The model under review builds one solid part; all positions refer to its coordinate system, in mm. Face numbers are marked on the shaded views. A direction names the side the tool comes from. Round coordinates to 2 decimals unless told otherwise and drop trailing zeros. Write each loop counter-clockwise with the first axis right and the second up, starting at its lowest first coordinate (ties: lowest second). Pieces come first, ordered by that corner, then holes. Notation, with made-up numbers: M 49.5,20.5 L 91.5,20.5 A31 cw 91.5,56.5 Z; hole C 45.25,-15.75 d9. An arc over 180 degrees is marked long. One line per item, written item: value. Start each with the question number.
1) Take a section at A-A, the plane x = 30. Write out the cut boundary in (y, z).
2) Wall thickness on probe 1 along Y at (x, z) = (0, 1.5); probe 2 along X at (y, z) = (-17.5, 0.5); probe 3 along X at (y, z) = (41.5, 0.75): over which ranges is each line inside the solid? List them lowest first.
3) Tool access review of the marked faces 4 and 5: name each direction out of +Z, -Z, +X, -X, +Y, -Y from which nothing blocks a thin tool from reaching the whole face with its end or side.
4) Take a section at B-B, the plane y = 20. Write out the cut boundary in (x, z), and give its area (3 significant figures).
5) Mouldability with a two-part tool opening along Y and no side actions: class the marked faces 1, 2 and 3 as +Y half, -Y half, draft (parallel to the pull), parting line (faces both ways), or undercut.
6) For P1, Ø2.5, axis at x = -66.82, y = 3.94, coming from the +Z side; P2, Ø4, axis at y = 53.5, z = 6.5, coming from the +X side; P3, Ø1.5, axis at x = 48.5, y = -28.5, coming from the +Z side; P4, Ø4, axis at x = 45, z = 4.5, coming from the -Y side, all flat-tipped, find the tip position at first contact; note any pin that passes through.
from build123d import *

# Parameters (mm, degrees)
BOSS_EXTRUDE1_DEPTH = 8
SKETCH2_R           = 2.25
CUT_EXTRUDE1_DEPTH  = 28
FILLET1_R           = 10
SKETCH5_R           = 1.65
CUT_EXTRUDE3_DEPTH  = 45
SKETCH10_R          = 4
CUT_EXTRUDE4_DEPTH  = 5
CUT_EXTRUDE5_DEPTH  = 10
CHAMFER1_SIZE       = 8.908764189
CHAMFER1_SIZE_2     = 10
CHAMFER1_SIZE_3     = 8.898783464
SKETCH12_R          = 10
CUT_EXTRUDE6_DEPTH  = 25.5
SKETCH13_R          = 1.65
CUT_EXTRUDE7_DEPTH  = 10
SKETCH14_R          = 2.55
CUT_EXTRUDE8_DEPTH  = 2.3
FILLET2_R           = 3
SKETCH15_R          = 2.5
CUT_EXTRUDE9_DEPTH  = 3


with BuildPart() as part:
    # Sketch1 → Boss-Extrude1 (new body)
    with BuildSketch(Plane.XY):
        Polygon((40, 69.282032303), (-40, 69.282032303), (-80, 0), (-40, -69.282032303), (40, -69.282032303), (80, 0), align=None)
    extrude(amount=BOSS_EXTRUDE1_DEPTH)

    # Sketch2 → Cut-Extrude1 (cut)
    with BuildSketch(Plane.XY.offset(8)):
        with Locations((-36.81613895, 55.896823885)):
            Circle(SKETCH2_R)
        with Locations((-66.81613895, 3.935299658)):
            Circle(SKETCH2_R)
        with Locations((36.81613895, 55.896823885)):
            Circle(SKETCH2_R)
        with Locations((66.81613895, 3.935299658)):
            Circle(SKETCH2_R)
        with Locations((30, -59.832123543)):
            Circle(SKETCH2_R)
        with Locations((-30, -59.832123543)):
            Circle(SKETCH2_R)
    extrude(amount=-CUT_EXTRUDE1_DEPTH, mode=Mode.SUBTRACT)

    # Fillet1
    fillet1_edges = [part.edges().sort_by_distance(p)[0] for p in [
        (80, 0, 4),
        (40, -69.282032303, 4),
        (-40, -69.282032303, 4),
        (-80, 0, 4),
        (-40, 69.282032303, 4),
        (40, 69.282032303, 4),
    ]]
    fillet(fillet1_edges, radius=FILLET1_R)

    # Sketch5 → Cut-Extrude3 (cut)
    with BuildSketch(Plane.XY.offset(8)):
        with Locations((0, 55)):
            Circle(SKETCH5_R)
        with Locations((47.631397208, -27.5)):
            Circle(SKETCH5_R)
        with Locations((-47.631397208, -27.5)):
            Circle(SKETCH5_R)
    extrude(amount=-CUT_EXTRUDE3_DEPTH, mode=Mode.SUBTRACT)

    # Sketch10 → Cut-Extrude4 (cut)
    with BuildSketch(Plane(origin=(0, 0, 0), x_dir=(-1, 0, 0), z_dir=(0, 0, -1))):
        with Locations((-30, -59.832123543)):
            Circle(SKETCH10_R)
        with Locations((-66.81613895, 3.935299658)):
            Circle(SKETCH10_R)
        with Locations((-36.81613895, 55.896823885)):
            Circle(SKETCH10_R)
        with Locations((36.81613895, 55.896823885)):
            Circle(SKETCH10_R)
        with Locations((66.81613895, 3.935299658)):
            Circle(SKETCH10_R)
        with Locations((30, -59.832123543)):
            Circle(SKETCH10_R)
    extrude(amount=-CUT_EXTRUDE4_DEPTH, mode=Mode.SUBTRACT)

    # Sketch11 → Cut-Extrude5 (cut)
    with BuildSketch(Plane(origin=(0, 0, 0), x_dir=(-1, 0, 0), z_dir=(0, 0, -1))):
        with BuildLine():
            Line((-6.556209751, -49.568297466), (-6.556209751, -6.628815438))
            Line((-6.556209751, -6.628815438), (-49.558640073, -6.628815438))
            ThreePointArc((-49.558640073, -6.628815438), (-35.329433507, -35.381225644), (-6.556209751, -49.568297466))
        make_face()
        with BuildLine():
            Line((6.556209751, -49.568297466), (6.556209751, -6.628815438))
            Line((6.556209751, -6.628815438), (49.558640073, -6.628815438))
            ThreePointArc((49.558640073, -6.628815438), (35.329433507, -35.381225644), (6.556209751, -49.568297466))
        make_face()
        with BuildLine():
            Line((-49.558640073, 6.628815438), (-6.556209751, 6.628815438))
            Line((-6.556209751, 6.628815438), (-6.556209751, 49.568297466))
            ThreePointArc((-6.556209751, 49.568297466), (-35.329433507, 35.381225644), (-49.558640073, 6.628815438))
        make_face()
        with BuildLine():
            Line((6.556209751, 6.628815438), (49.558640073, 6.628815438))
            ThreePointArc((49.558640073, 6.628815438), (35.329433507, 35.381225644), (6.556209751, 49.568297466))
            Line((6.556209751, 49.568297466), (6.556209751, 6.628815438))
        make_face()
    extrude(amount=-CUT_EXTRUDE5_DEPTH, mode=Mode.SUBTRACT)

    # Chamfer1
    # the kernel refuses this chamfer: 10, 8.908764189, 8.898783464 mm, written as the material it adds along each edge
    with BuildSketch(Plane(origin=(-6.556209751, 49.568297466, 0), x_dir=(-0.9751121847064436, -0.22171203674367113, 0), z_dir=(0, 0, 1)), Plane(origin=(6.556209751, -49.568297466, 0), x_dir=(0.9751121847064436, 0.22171203674367113, 0), z_dir=(0, 0, 1))) as chamfer1_piece_1:
        with BuildLine():
            Line((9.19369635, 0), (CHAMFER1_SIZE * 0.221712036732, CHAMFER1_SIZE * 0.975112184657))
            Line((CHAMFER1_SIZE * 0.221712036732, CHAMFER1_SIZE * 0.975112184657), (0, 0))
            ThreePointArc((0, 0), (4.724816594, -0.211594789), (9.19369635, 0))
        make_face()
    extrude(amount=8)
    with BuildSketch(Plane(origin=(-49.558640073, 6.628815438, 0), x_dir=(0.2152729733414999, 0.9765539139999951, 0), z_dir=(0, 0, 1)), Plane(origin=(49.558640073, -6.628815438, 0), x_dir=(-0.2152729733414999, -0.9765539139999951, 0), z_dir=(0, 0, 1))) as chamfer1_piece_2:
        with BuildLine():
            Line((8.390480284, 0), (CHAMFER1_SIZE_2 * 0.215272973341, -CHAMFER1_SIZE_2 * 0.976553914))
            Line((CHAMFER1_SIZE_2 * 0.215272973341, -CHAMFER1_SIZE_2 * 0.976553914), (0, 0))
            ThreePointArc((0, 0), (4.30291799, 0.17619531), (8.390480284, 0))
        make_face()
    extrude(amount=8)
    with BuildSketch(Plane(origin=(-6.556209751, 6.628815438, 0), x_dir=(-1, 0, 0), z_dir=(0, 0, 1)), Plane(origin=(-6.556209751, -6.628815438, 0), x_dir=(0, -1, 0), z_dir=(0, 0, 1)), Plane(origin=(6.556209751, -6.628815438, 0), x_dir=(1, 0, 0), z_dir=(0, 0, 1)), Plane(origin=(6.556209751, 6.628815438, 0), x_dir=(0, 1, 0), z_dir=(0, 0, 1))) as chamfer1_piece_3:
        Polygon((CHAMFER1_SIZE_2, 0), (0, -CHAMFER1_SIZE_2), (0, 0), align=None)
    extrude(amount=8)
    with BuildSketch(Plane(origin=(-49.558640073, -6.628815438, 0), x_dir=(0.22314024310111003, -0.9747863519298869, 0), z_dir=(0, 0, 1))) as chamfer1_piece_4:
        with BuildLine():
            Line((9.19369635, 0), (CHAMFER1_SIZE_3 * 0.223140243107, CHAMFER1_SIZE_3 * 0.974786351955))
            Line((CHAMFER1_SIZE_3 * 0.223140243107, CHAMFER1_SIZE_3 * 0.974786351955), (0, 0))
            ThreePointArc((0, 0), (4.724816594, -0.211594789), (9.19369635, 0))
        make_face()
    extrude(amount=8)
    with BuildSketch(Plane(origin=(-6.556209751, -49.568297466, 0), x_dir=(-0.9768521989550364, 0.21391536035710523, 0), z_dir=(0, 0, 1))) as chamfer1_piece_5:
        with BuildLine():
            Line((8.397944605, 0), (CHAMFER1_SIZE_2 * 0.213915360357, -CHAMFER1_SIZE_2 * 0.976852198955))
            Line((CHAMFER1_SIZE_2 * 0.213915360357, -CHAMFER1_SIZE_2 * 0.976852198955), (0, 0))
            ThreePointArc((0, 0), (4.306885367, 0.176509198), (8.397944605, 0))
        make_face()
    extrude(amount=8)
    with BuildSketch(Plane(origin=(6.556209751, 49.568297466, 0), x_dir=(0, -1, 0), z_dir=(0, 0, 1))) as chamfer1_piece_6:
        with BuildLine():
            Line((CHAMFER1_SIZE_2, 0), (1.796449346, 8.203550654))
            ThreePointArc((1.796449346, 8.203550654), (0.748885537, 4.24494847), (0, 0))
            Line((0, 0), (CHAMFER1_SIZE_2, 0))
        make_face()
    extrude(amount=8)
    with BuildSketch(Plane(origin=(49.558640073, 6.628815438, 0), x_dir=(-1, 0, 0), z_dir=(0, 0, 1))) as chamfer1_piece_7:
        with BuildLine():
            Line((CHAMFER1_SIZE_3, 0), (2.051483639, -8.961889726))
            ThreePointArc((2.051483639, -8.961889726), (0.848037011, -4.652902044), (0, 0))
            Line((0, 0), (CHAMFER1_SIZE_3, 0))
        make_face()
    extrude(amount=8)

    # Sketch12 → Cut-Extrude6 (cut)
    with BuildSketch(Plane(origin=(0, 0, 0), x_dir=(-1, 0, 0), z_dir=(0, 0, -1))):
        Circle(SKETCH12_R)
    extrude(amount=-CUT_EXTRUDE6_DEPTH, mode=Mode.SUBTRACT)

    # Sketch13 → Cut-Extrude7 (cut)
    with BuildSketch(Plane(origin=(0, 0, 0), x_dir=(-1, 0, 0), z_dir=(0, 0, -1))):
        with Locations((0, 30)):
            Circle(SKETCH13_R)
        with Locations(Location((0, -30, 0), (0, 0, 180))):
            Circle(SKETCH13_R)
    extrude(amount=-CUT_EXTRUDE7_DEPTH, mode=Mode.SUBTRACT)

    # Sketch14 → Cut-Extrude8 (cut)
    with BuildSketch(Plane(origin=(0, 0, 0), x_dir=(-1, 0, 0), z_dir=(0, 0, -1))):
        with Locations((0, -30)):
            Circle(SKETCH14_R)
        with Locations((0, 30)):
            Circle(SKETCH14_R)
    extrude(amount=-CUT_EXTRUDE8_DEPTH, mode=Mode.SUBTRACT)

    # Fillet2
    fillet2_edges = [part.edges().sort_by_distance(p)[0] for p in [
        (-6.556209751, -39.568297466, 4),
        (-6.556209751, -16.628815438, 4),
        (-40.659856609, -6.628815438, 4),
        (-16.556209751, -6.628815438, 4),
        (-14.759760405, -47.77184812, 4),
        (-47.507156434, -15.590705164, 4),
        (6.556209751, -16.628815438, 4),
        (6.556209751, -40.659533278, 4),
        (47.752396435, -14.8225718, 4),
        (15.521095085, -47.529944323, 4),
        (39.558640073, -6.628815438, 4),
        (16.556209751, -6.628815438, 4),
        (47.507156434, 15.590705164, 4),
        (14.759760405, 47.77184812, 4),
        (6.556209751, 16.628815438, 4),
        (6.556209751, 39.568297466, 4),
        (16.556209751, 6.628815438, 4),
        (40.659856609, 6.628815438, 4),
        (-15.521095085, 47.529944323, 4),
        (-47.752396435, 14.8225718, 4),
        (-16.556209751, 6.628815438, 4),
        (-39.558640073, 6.628815438, 4),
        (-6.556209751, 40.659533278, 4),
        (-6.556209751, 16.628815438, 4),
    ]]
    fillet(fillet2_edges, radius=FILLET2_R)

    # Sketch15 → Cut-Extrude9 (cut)
    with BuildSketch(Plane.XY.offset(8)):
        with Locations((-47.631397208, -27.5)):
            Circle(SKETCH15_R)
        with Locations((0, 55)):
            Circle(SKETCH15_R)
        with Locations((47.631397208, -27.5)):
            Circle(SKETCH15_R)
    extrude(amount=-CUT_EXTRUDE9_DEPTH, mode=Mode.SUBTRACT)


solid = part.part
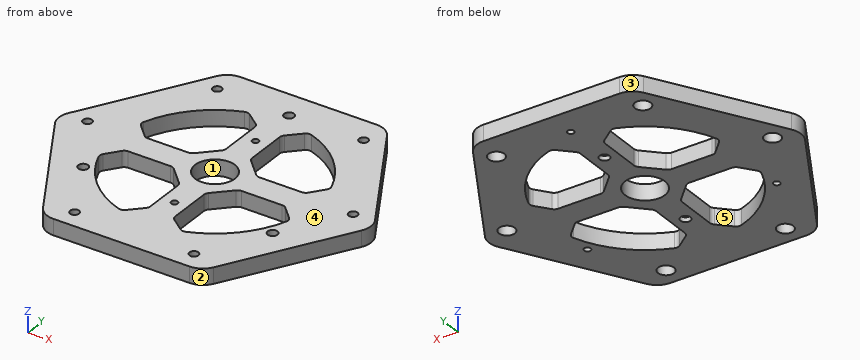
Checked values:
1. outline: M -69.28,0 L -63.83,0 L -63.83,5 L -62.08,5 L -62.08,8 L -69.28,8 Z; M -57.58,5 L -55.83,5 L -55.83,0 L -40,0 L -40,8 L -57.58,8 Z; M -6.63,0 L 6.63,0 L 6.63,8 L -6.63,8 Z; M 40,0 L 69.28,0 L 69.28,8 L 40,8 Z
2. probe 1: y = -69.28 to -32.55, -27.45 to -10, 10 to 27.45, 32.55 to 53.35, 56.65 to 69.28
2. probe 2: x = -69.9 to -46.84, -6.58 to 6.58, 46.84 to 69.9
2. probe 3: x = -56.04 to -27.89, -7.66 to 8.49, 27.89 to 56.04
3. face 4: +Z, +X, -X, +Y, -Y
3. face 5: +Z, -Z
4. outline: M -68.45,0 L -45.83,0 L -45.83,8 L -68.45,8 Z; M -6.56,0 L 6.56,0 L 6.56,8 L -6.56,8 Z; M 45.83,0 L 68.45,0 L 68.45,8 L 45.83,8 Z
4. area: 467 mm2
5. face 1: undercut
5. face 2: -Y half
5. face 3: +Y half
6. P1: passes through
6. P2: stops at x = 50.27
6. P3: stops at z = 5
6. P4: stops at y = -64.09
